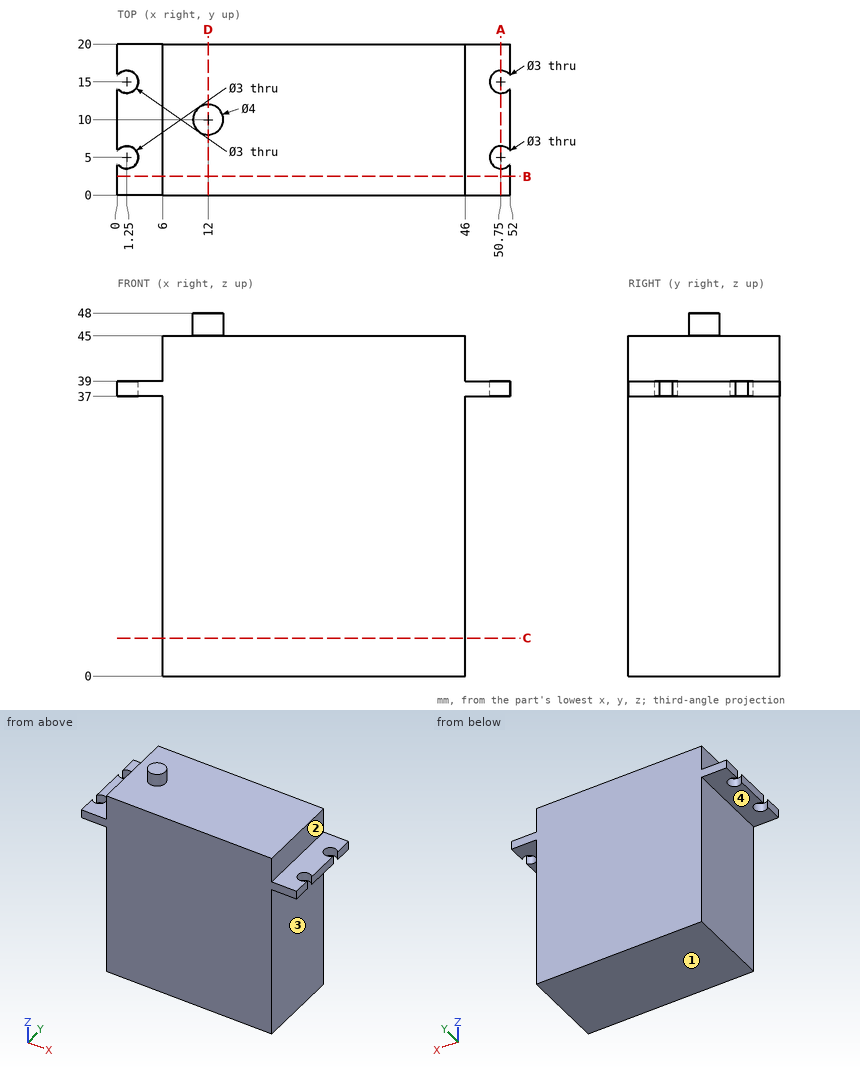
Answer from the drawing. Dimensions are ordinates in mm from the lowest x, y and z of the part. A direction names the side the tool comes from. Coordinates: 2 decimals unless noted, no trailing zeros. Loops run counter-clockwise (first coordinate to the right, second up) from the corner with the lowest first, then second, coordinate; pieces in that order, holes last. Notation, with made-up numbers: (18, 52) - (38, 52) arc R18 cw to (38, 74) - close; hole circle Ø6 at (14.5, 87). An arc over 180 degrees is marked (long way). Use a Markdown table: item, result.
Item 1: Find section C-C, the plane z = 5. Determine the outline of the cut face in (x, y), and give its area (3 significant figures).
Evaluation:
| item | result |
|---|---|
| outline | (6, 0) - (46, 0) - (46, 20) - (6, 20) - close |
| area | 800 mm2 |
Item 2: Find section B-B, the plane y = 2.5. Determine the outline of the cut face in (x, z).
Evaluation:
| item | result |
|---|---|
| outline | (0, 37) - (6, 37) - (6, 0) - (46, 0) - (46, 37) - (52, 37) - (52, 39) - (46, 39) - (46, 45) - (6, 45) - (6, 39) - (0, 39) - close |
Item 3: Given pin 1 Ø3 at (x, y) = (48, 9.5) entering from -Z; pin 2 Ø6 at (y, z) = (8.5, 24.5) entering from -X; pin 3 Ø8 at (x, y) = (6.5, 7.5) entering from +Z, each flat-ended and moving along its own axis, determine where each tip first touches the part or whether it passes through.
Evaluation:
| item | result |
|---|---|
| pin 1 | stops at z = 37 |
| pin 2 | stops at x = 6 |
| pin 3 | stops at z = 45 |
Item 4: Consider probe 1 along Y at (x, z) = (50.75, 37.4); probe 2 along Z at (x, y) = (14.5, 3); probe 3 along X at (y, z) = (5, 37.6). Determine where each line is inside the solid, lowest interval first. Write a range as from..to.
Evaluation:
| item | result |
|---|---|
| probe 1 | y = 0..3.5, 6.5..13.5, 16.5..20 |
| probe 2 | z = 0..45 |
| probe 3 | x = 2.75..49.25 |
Item 5: Find section D-D, the plane x = 12. Determine the outline of the cut face in (y, z), and give its area (3 significant figures).
Evaluation:
| item | result |
|---|---|
| outline | (0, 0) - (20, 0) - (20, 45) - (12, 45) - (12, 48) - (8, 48) - (8, 45) - (0, 45) - close |
| area | 912 mm2 |
Item 6: Find section A-A, the plane x = 50.75. Determine the outline of the cut face in (y, z).
Evaluation:
| item | result |
|---|---|
| outline | (0, 37) - (3.5, 37) - (3.5, 39) - (0, 39) - close; (6.5, 37) - (13.5, 37) - (13.5, 39) - (6.5, 39) - close; (16.5, 37) - (20, 37) - (20, 39) - (16.5, 39) - close |
Item 7: For the marked faces 1, 2, 3 and 4, determine the directions among +Z, -Z, +X, -X, +Y, -Y from which every point of the face is accessible in a straight line to the end or side of a thin tool.
Evaluation:
| item | result |
|---|---|
| face 1 | -Z, +X, -X, +Y, -Y |
| face 2 | +Z, +X, +Y, -Y |
| face 3 | -Z, +X, +Y, -Y |
| face 4 | -Z, -X, +Y, -Y |
